Autodesk Inventor part; units mm, degrees
ref_plane "XZ Plane" through (0, 0, 0) normal (0, 1, 0) x (-1, 0, 0)
ref_plane "XY Plane" through (0, 0, 0) normal (0, 0, 1) x (1, 0, 0)
sketch "Sketch1" plane through (0, 0, 0) normal (0, 1, 0) x (-1, 0, 0)
  line L0 (47.625, 47.625) -> (-47.625, 47.625)
  line L1 (-47.625, 47.625) -> (-47.625, -47.625)
  line L2 (-47.625, -47.625) -> (47.625, -47.625)
  line L3 (47.625, -47.625) -> (47.625, 47.625)
  line L4 (47.625, 47.625) -> (-47.625, -47.625) construction
  line L5 (-47.625, 47.625) -> (47.625, -47.625) construction
  point P0 (0, 0)
  dimension "d0" = 95.25
  dimension "d1" = 95.25
extrude "Extrusion1" add sketch "Sketch1" along normal blind 6.35
sketch "Sketch2" plane through (-47.625, 0, 47.625) normal (0, 0, 1) x (1, 0, 0)
  line L0 (0, 6.35) -> (95.25, 6.35)
  line L1 (25.4, 6.35) -> (44.45, 6.35)
  line L2 (44.45, 6.35) -> (44.45, 50.8)
  line L3 (44.45, 50.8) -> (25.4, 50.8)
  line L4 (25.4, 50.8) -> (25.4, 6.35)
  line L5 (50.8, 6.35) -> (69.85, 6.35)
  line L6 (69.85, 6.35) -> (69.85, 50.8)
  line L7 (69.85, 50.8) -> (50.8, 50.8)
  line L8 (50.8, 50.8) -> (50.8, 6.35)
  line L9 (0, 0) -> (0, 6.35)
  line L10 (28.575, 9.525) -> (41.275, 9.525)
  line L11 (41.275, 9.525) -> (41.275, 47.625)
  line L12 (41.275, 47.625) -> (28.575, 47.625)
  line L13 (28.575, 47.625) -> (28.575, 9.525)
  line L14 (28.575, 9.525) -> (41.275, 47.625) construction
  line L15 (41.275, 9.525) -> (28.575, 47.625) construction
  line L16 (53.975, 9.525) -> (66.675, 9.525)
  line L17 (66.675, 9.525) -> (66.675, 47.625)
  line L18 (66.675, 47.625) -> (53.975, 47.625)
  line L19 (53.975, 47.625) -> (53.975, 9.525)
  line L20 (53.975, 9.525) -> (66.675, 47.625) construction
  line L21 (66.675, 9.525) -> (53.975, 47.625) construction
  point P0 (47.625, 0)
  point P1 (34.925, 28.575)
  point P2 (60.325, 28.575)
  dimension "d4" = 19.05
  dimension "d5" = 44.45
  dimension "d6" = 6.35
  dimension "d7" = 25.4
  dimension "d8" = 3.175
  dimension "d9" = 3.175
  dimension "d10" = 3.175
  dimension "d11" = 3.175
  dimension "d12" = 3.175
  dimension "d13" = 3.175
extrude "Extrusion2" add sketch "Sketch2" against normal blind 95.25
sketch "Sketch3" plane through (-22.225, 50.8, 47.625) normal (0, 1, 0) x (1, 0, 0)
  line L0 (0, 0) -> (0, 95.25)
  line L1 (0, 0) -> (44.45, 0)
  line L2 (44.45, 0) -> (44.45, 95.25)
  line L3 (44.45, 95.25) -> (0, 95.25)
  line L4 (0, 95.25) -> (0, 0)
  point P0 (22.225, 47.625)
extrude "Extrusion3" add sketch "Sketch3" along normal blind 25.4
sketch "Sketch4" plane through (0, 6.35, 0) normal (0, 1, 0) x (1, 0, 0)
  line L0 (-47.625, -47.625) -> (47.625, -47.625) construction
  line L1 (-34.925, -47.625) -> (-34.925, 47.625) construction
  line L2 (-47.625, 47.625) -> (-47.625, -47.625)
  line L3 (34.925, -47.625) -> (34.925, 47.625) construction
  line L4 (47.625, -47.625) -> (47.625, 47.625) construction
  point P0 (0, 0)
  point P1 (-34.925, -23.8125)
  point P2 (-34.925, 0)
  point P3 (-34.925, 23.8125)
  dimension "d18" = 12.7
  dimension "d19" = 12.7
  dimension "d20" = 23.8125
  dimension "d21" = 23.8125
  dimension "d22" = 23.8125
hole "Hole1" at (-34.925, 6.35, 23.8125) at (-34.925, 6.35, 0) at (-34.925, 6.35, -23.8125) direction (0, -1, 0) diameter 6.7564 end through all
mirror "Mirror1" about plane through (0, 0, 0) normal (1, 0, 0) of "Hole1"
equation "\"d0\" = width"
equation "\"d1\" = length"
equation "\"d2\" = thickness"
equation "\"d4\" = tubeWidth"
equation "\"d5\" = tubeLength"
equation "\"d8\" = tubeWallThickness"
equation "\"d9\" = tubeWallThickness"
equation "\"d10\" = tubeWallThickness"
equation "\"d11\" = tubeWallThickness"
equation "\"d12\" = tubeWallThickness"
equation "\"d13\" = tubeWallThickness"
equation "\"d14\" = length"
equation "\"length\" = 95.25"
equation "\"width\" = 95.25"
equation "\"thickness\" = 6.35"
equation "\"tubeLength\" = 44.45"
equation "\"tubeWidth\" = 19.05"
equation "\"tubeWallThickness\" = 3.175"
properties part number "SupportForMotorMountV02"
Geometry: final body of the model. Coordinates: model frame, mm. A direction names the side the tool comes from. Give positions to 0.01 mm unless a question says otherwise; leave off trailing zeros. Loops run counter-clockwise (first coordinate to the right, second up) from the corner with the lowest first, then second, coordinate; pieces in that order, holes last. Notation, with made-up numbers: (8, 89.5) -> (59, 89.5) arc R33 ccw to (59, 126.5) -> close; hole circle Ø4 at (46, 65). An arc over 180 degrees is marked (long way). Use one line per item in the form item = value.
Item 1: Section query A-A on z = 0. Output: boundary loops of the cut face in (x, y) (3 decimals), and give its area (3 significant figures).
A:
outline = (-47.625, 0) -> (-38.303, 0) -> (-38.303, 6.35) -> (-47.625, 6.35) -> close; (-31.547, 0) -> (31.547, 0) -> (31.547, 6.35) -> (22.225, 6.35) -> (22.225, 76.2) -> (-22.225, 76.2) -> (-22.225, 6.35) -> (-31.547, 6.35) -> close; (38.303, 0) -> (47.625, 0) -> (47.625, 6.35) -> (38.303, 6.35) -> close; hole (-19.05, 9.525) -> (-6.35, 9.525) -> (-6.35, 47.625) -> (-19.05, 47.625) -> close; hole (-3.175, 6.35) -> (3.175, 6.35) -> (3.175, 50.8) -> (-3.175, 50.8) -> close; hole (6.35, 9.525) -> (19.05, 9.525) -> (19.05, 47.625) -> (6.35, 47.625) -> close
area = 2,370 mm^2
Item 2: Access query for faces 5 (the face through (-22.225, 41, 1)), 6 (the face through (-6.35, 28, 1)), 7 (the face through (41, 6.35, 1)), 8 (the face through (1, 54, -47.625)). Directions: +Z, -Z, +X, -X, +Y, -Y. A direction counts if a zero-diameter tool reaches every point of the face in a straight line with its end or side. Return the directions, or none.
A:
face_5 = +Z, -Z, -X, +Y
face_6 = +Z, -Z
face_7 = +Z, -Z, +X, +Y
face_8 = -Z, +X, -X, +Y, -Y
Item 3: Section query C-C on y = 14. Output: boundary loops of the cut face in (x, z) (3 decimals).
A:
outline = (-22.225, -47.625) -> (-19.05, -47.625) -> (-19.05, 47.625) -> (-22.225, 47.625) -> close; (-6.35, -47.625) -> (-3.175, -47.625) -> (-3.175, 47.625) -> (-6.35, 47.625) -> close; (3.175, -47.625) -> (6.35, -47.625) -> (6.35, 47.625) -> (3.175, 47.625) -> close; (19.05, -47.625) -> (22.225, -47.625) -> (22.225, 47.625) -> (19.05, 47.625) -> close
Item 4: Line query: probe 1 along X at (y, z) = (21.5, 7) (3 decimals); probe 2 along X at (y, z) = (1.75, 0) (3 decimals); probe 3 along Y at (x, z) = (-8.5, 35) (3 decimals). Output: solid intervals per line, ascending.
A:
probe_1 = -22.225 to -19.05, -6.35 to -3.175, 3.175 to 6.35, 19.05 to 22.225
probe_2 = -47.625 to -38.303, -31.547 to 31.547, 38.303 to 47.625
probe_3 = 0 to 9.525, 47.625 to 76.2
Item 5: Section query B-B on x = -13. Output: boundary loops of the cut face in (y, z) (3 decimals).
A:
outline = (0, -47.625) -> (9.525, -47.625) -> (9.525, 47.625) -> (0, 47.625) -> close; (47.625, -47.625) -> (76.2, -47.625) -> (76.2, 47.625) -> (47.625, 47.625) -> close
Item 6: Section query D-D on x = 37. Output: boundary loops of the cut face in (y, z) (3 decimals).
A:
outline = (0, -47.625) -> (6.35, -47.625) -> (6.35, -26.478) -> (0, -26.478) -> close; (0, -21.147) -> (6.35, -21.147) -> (6.35, -2.666) -> (0, -2.666) -> close; (0, 2.666) -> (6.35, 2.666) -> (6.35, 21.147) -> (0, 21.147) -> close; (0, 26.478) -> (6.35, 26.478) -> (6.35, 47.625) -> (0, 47.625) -> close
Item 7: Draft query along Z for faces 1 (the face through (0, 50.8, -1)), 2 (the face through (-37.774, 3.131, 25.629)), 3 (the face through (-1, 54, 47.625)), 4 (the face through (-37.774, 3.131, -21.996)). Return one class per face: pulls with the +Z half, pulls with the -Z half, needs draft (parallel to the pull), parting line crosses it, or undercut.
A:
face_1 = needs draft
face_2 = undercut
face_3 = pulls with the +Z half
face_4 = undercut
Item 8: Pin query (flat end, axial travel): P1, Ø4, axis at x = -34.92, z = -23.81, coming from the -Y side; P2, Ø5, axis at y = 67, z = 19.5, coming from the -X side (3 decimals); P3, Ø1, axis at y = 40, z = 0.5, coming from the +X side (3 decimals); P4, Ø9, axis at x = 34.92, z = -23.81, coming from the +Y side. Return the tip coordinate at first contact, or that it passes through.
A:
P1 = through
P2 = -22.225
P3 = 22.225
P4 = 6.35
